Answer from the drawing. Dimensions are ordinates in mm from the lowest x, y and z of the part. A direction names the side the tool comes from. Round coordinates to 2 decimals unless told otherwise and drop trailing zeros. Order: outer loops, then holes, each group sorted by start corner. A loop starts at its lowest first (then second) coordinate and runs counter-clockwise, first axis right, second up.
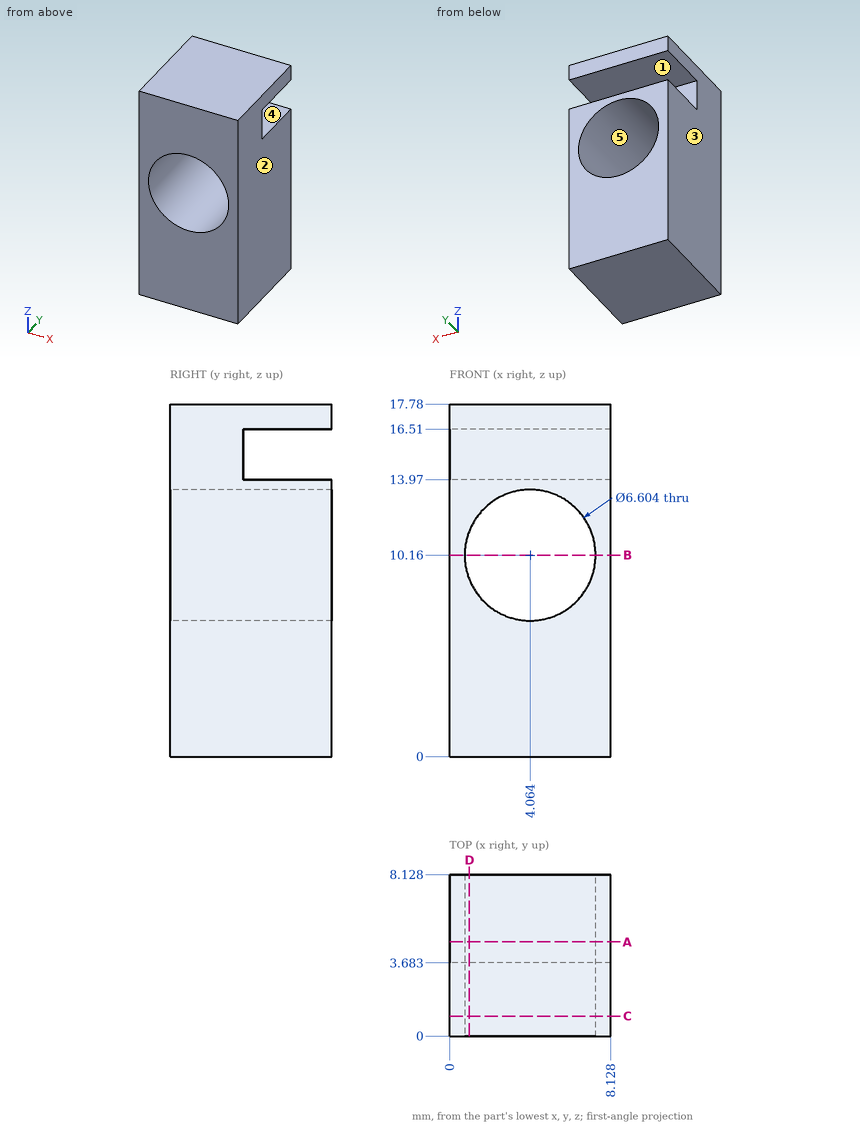
Q1. Flat-ended cylindrical pins translate along their axes: pin 1 (0.8 mm diameter, centred on x = 5, z = 15, fed in from +Y); pin 2 (2 mm diameter, centred on x = 5, z = 11, fed in from -Y). Find the tip coordinate at first contact, or state that the pin passes through.
Outcome:
pin 1: stops at y = 3.68
pin 2: passes through
Q2. For the marked faces 1 and 2, determine the directions among +Z, -Z, +X, -X, +Y, -Y from which every point of the face is accessible in a straight line to the end or side of a thin tool.
Outcome:
face 1: +X, -X, +Y
face 2: +Z, -Z, +X, +Y, -Y
Q3. A cutting plane is placed at C-C, the plane y = 1. Give the vertices of the cut face in (x, z), plus the area to 3 significant figures.
Outcome:
outline: (0, 0) - (8.13, 0) - (8.13, 17.78) - (0, 17.78) - close; hole circle Ø6.6 at (4.06, 10.16)
area: 110 mm2
Q4. A cutting plane is placed at B-B, the plane z = 10.16. Give the vertices of the cut face in (x, y).
Outcome:
outline: (0, 0) - (0.76, 0) - (0.76, 8.13) - (0, 8.13) - close; (7.37, 0) - (8.13, 0) - (8.13, 8.13) - (7.37, 8.13) - close
Q5. For a pull along X with two mould halves and no side action, classify the marked faces 3, 4 and 5 as released by +X, released by -X, zero draft, split by the parting line, or undercut.
Outcome:
face 3: released by -X
face 4: zero draft
face 5: undercut
Q6. Straight lines are drawn through the part: probe 1 along Z at (x, y) = (4, 7); probe 2 along Z at (x, y) = (3.5, 5.25); probe 3 along Z at (x, y) = (7.75, 7.5). For each, find the intervals that lie inside material, in ascending order.
Outcome:
probe 1: z = 0 to 6.86, 13.46 to 13.97, 16.51 to 17.78
probe 2: z = 0 to 6.91, 13.41 to 13.97, 16.51 to 17.78
probe 3: z = 0 to 13.97, 16.51 to 17.78
Q7. A cutting plane is placed at D-D, the plane x = 1. Give the vertices of the cut face in (y, z).
Outcome:
outline: (0, 0) - (8.13, 0) - (8.13, 8.93) - (0, 8.93) - close; (0, 11.39) - (8.13, 11.39) - (8.13, 13.97) - (3.68, 13.97) - (3.68, 16.51) - (8.13, 16.51) - (8.13, 17.78) - (0, 17.78) - close
Q8. A cutting plane is placed at A-A, the plane y = 4.75. Give the vertices of the cut face in (x, z).
Outcome:
outline: (0, 0) - (8.13, 0) - (8.13, 13.97) - (0, 13.97) - close; (0, 16.51) - (8.13, 16.51) - (8.13, 17.78) - (0, 17.78) - close; hole circle Ø6.6 at (4.06, 10.16)
